Can you work these out from the drawing? Everything is in mm from the part's minimum corner. Give positions to 0.01 mm unless a question says otherwise; leave off trailing zeros. Write each loop counter-clockwise with the first axis right and the second up, starting at its lowest first coordinate (ties: lowest second). Pieces come first, ordered by that corner, then holes. Notation, with made-up numbers: (87, 37) -> (112, 37) arc R15 cw to (112, 51) -> close; hole circle Ø1 at (-22, 63). An arc over 180 degrees is marked (long way). Return JSON: item names as keys, results as strings.
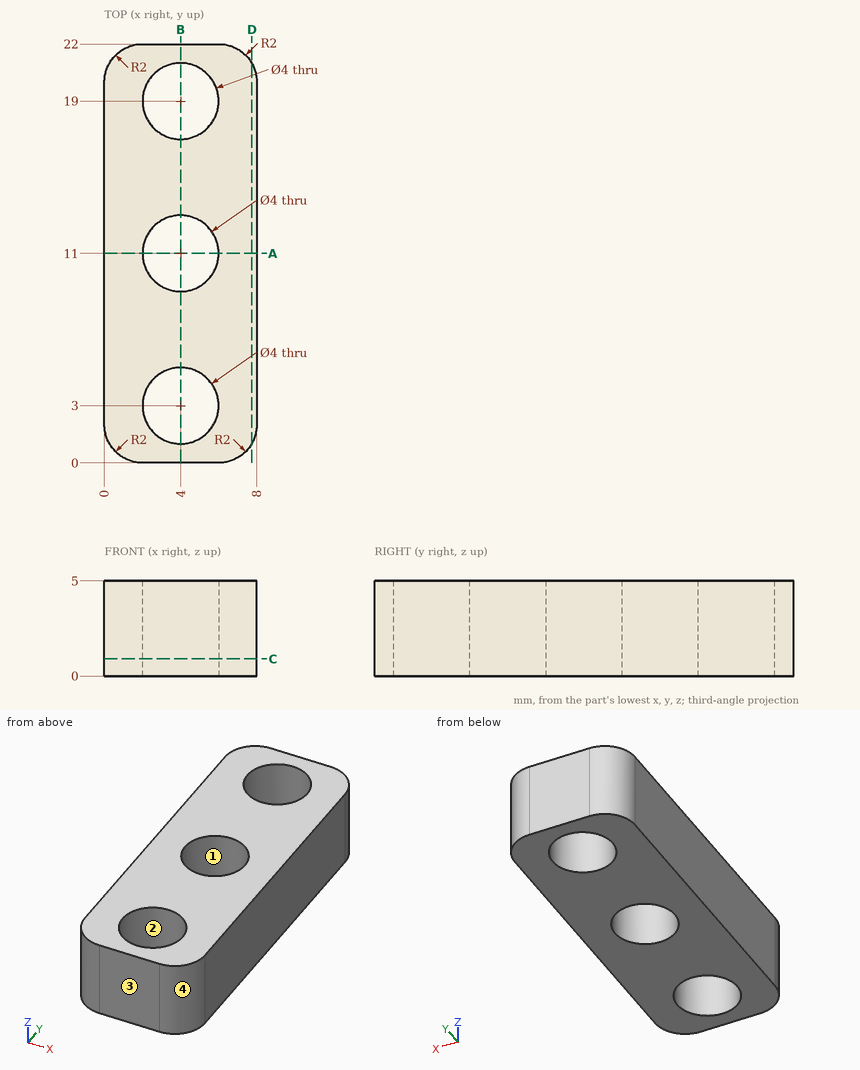
1. Suppose I cut it at D-D, the plane x = 7.75. List the corners of the cut face in (y, z) for me.
Taken from the geometry:
{"outline": "(1.03, 0) -> (20.97, 0) -> (20.97, 5) -> (1.03, 5) -> close"}
2. For pin 1 Ø2.5 at (x, y) = (4, 11) entering from -Z, with a flat end and sliding along its axis, tell me the tip position at first contact or that it passes through.
Taken from the geometry:
{"pin 1": "passes through"}
3. Suppose I cut it at A-A, the plane y = 11. List the corners of the cut face in (x, z) for me.
Taken from the geometry:
{"outline": "(0, 0) -> (2, 0) -> (2, 5) -> (0, 5) -> close; (6, 0) -> (8, 0) -> (8, 5) -> (6, 5) -> close"}
4. If we mould it in two halves opening along X, with no side actions, what happens to the marked faces 1, 2, 3 and 4? For each: released by +X, released by -X, zero draft, split by the parting line, or undercut.
Taken from the geometry:
{"face 1": "undercut", "face 2": "undercut", "face 3": "zero draft", "face 4": "released by +X"}
5. If I drill on line 1 (Y direction, x = 4, z = 3.35); line 2 (Y direction, x = 5.75, z = 1.25); line 3 (X direction, y = 19.75, z = 0.8), over which ranges is the centre line in solid material (lowest first)? Write a range as [from, to].
Taken from the geometry:
{"line 1": "y = [0, 1], [5, 9], [13, 17], [21, 22]", "line 2": "y = [0, 2.03], [3.97, 10.03], [11.97, 18.03], [19.97, 22]", "line 3": "x = [0, 2.15], [5.85, 8]"}
6. Suppose I cut it at B-B, the plane x = 4. List the corners of the cut face in (y, z) for me.
Taken from the geometry:
{"outline": "(0, 0) -> (1, 0) -> (1, 5) -> (0, 5) -> close; (5, 0) -> (9, 0) -> (9, 5) -> (5, 5) -> close; (13, 0) -> (17, 0) -> (17, 5) -> (13, 5) -> close; (21, 0) -> (22, 0) -> (22, 5) -> (21, 5) -> close"}
7. Suppose I cut it at C-C, the plane z = 0.9. List the corners of the cut face in (x, y) for me.
Taken from the geometry:
{"outline": "(0, 2) arc R2 ccw to (2, 0) -> (6, 0) arc R2 ccw to (8, 2) -> (8, 20) arc R2 ccw to (6, 22) -> (2, 22) arc R2 ccw to (0, 20) -> close; hole circle Ø4 at (4, 3); hole circle Ø4 at (4, 11); hole circle Ø4 at (4, 19)"}
